Check sheet for the drawn part. Datum: minimum x, y, z corner. Units: mm. A direction names the side the tool comes from. Round coordinates to 2 decimals unless told otherwise and drop trailing zeros. Loops run counter-clockwise (first coordinate to the right, second up) from the corner with the lowest first, then second, coordinate; pieces in that order, holes last. Notation, with made-up numbers: (64, -7) - (111, -7) arc R16 cw to (111, 19) - close; hole circle Ø2 at (-38, 64.25). An arc over 180 degrees is marked (long way). Use CSV: the item, a comma, the result in double quotes.
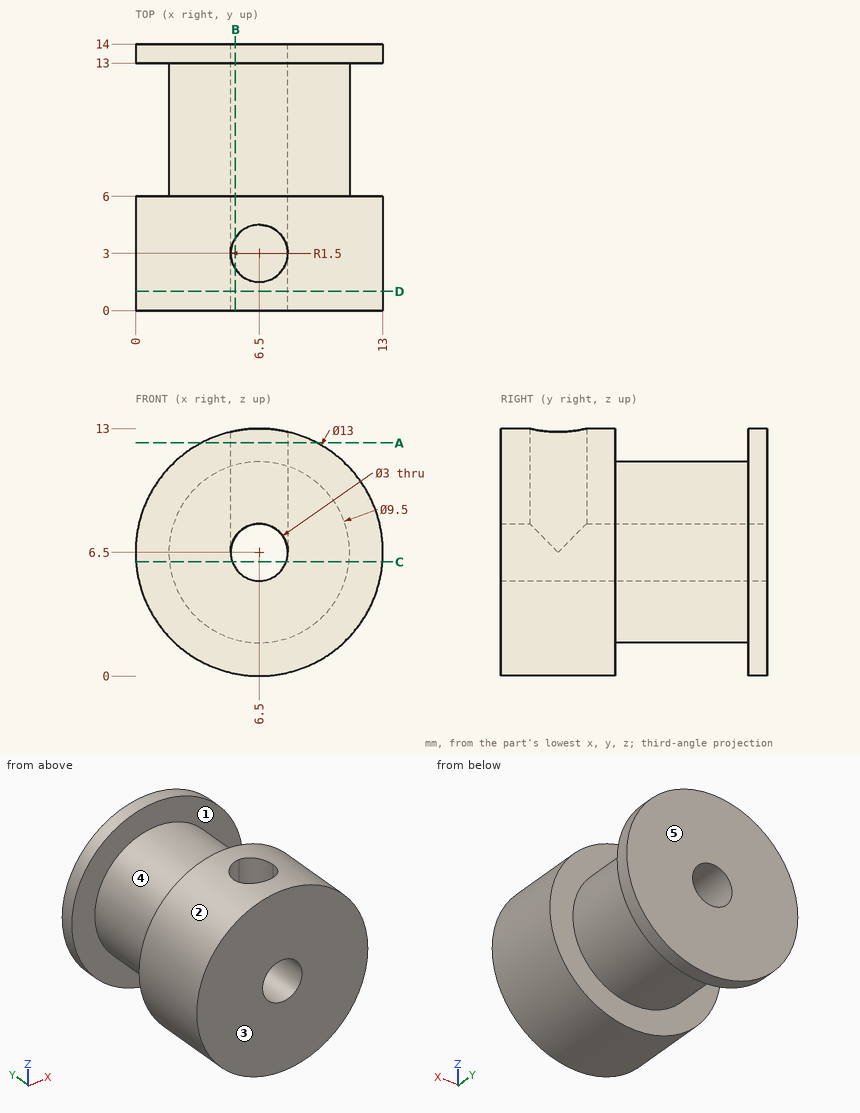
1) Gauge pin test, flat ends, axial feed: pin 1 Ø1.5 at (y, z) = (10.5, 8.5) entering from -X; pin 2 Ø1 at (y, z) = (6, 5.5) entering from -X. Record the tip position at first contact, or that the pin passes through.
Returned:
pin 1,"stops at x = 1.92"
pin 2,"stops at x = 0.02"
2) Cross-section at B-B, the plane x = 5.25. Record the cut outline in (y, z).
Returned:
outline,"(0, 0.12) - (6, 0.12) - (6, 1.92) - (13, 1.92) - (13, 0.12) - (14, 0.12) - (14, 5.67) - (0, 5.67) - close; (0, 7.33) - (2.17, 7.33) - (2.17, 12.88) - (0, 12.88) - close; (3.83, 7.33) - (14, 7.33) - (14, 12.88) - (13, 12.88) - (13, 11.08) - (6, 11.08) - (6, 12.88) - (3.83, 12.88) - close"
3) Cross-section at C-C, the plane z = 6. Record the cut outline in (x, y), then the cut area to 3 significant figures.
Returned:
outline,"(0.02, 0) - (5.09, 0) - (5.09, 14) - (0.02, 14) - (0.02, 13) - (1.78, 13) - (1.78, 6) - (0.02, 6) - close; (7.91, 0) - (12.98, 0) - (12.98, 6) - (11.22, 6) - (11.22, 13) - (12.98, 13) - (12.98, 14) - (7.91, 14) - close"
area,"117 mm²"
4) Cross-section at A-A, the plane z = 12.25. Record the cut outline in (x, y), then the cut area to 3 significant figures.
Returned:
outline,"(3.47, 0) - (9.53, 0) - (9.53, 6) - (3.47, 6) - close; (3.47, 13) - (9.53, 13) - (9.53, 14) - (3.47, 14) - close; hole circle Ø3 at (6.5, 3)"
area,"35.4 mm²"
5) Mould release check, pull along Y, two halves, no side actions. Record for the marked faces 3, 4 and 5: +Y half, -Y half, draft (parallel to the pull), parting line (faces both ways), or undercut.
Returned:
face 3,"-Y half"
face 4,"undercut"
face 5,"+Y half"
6) Access from +Z, -Z, +X, -X, +Y, -Y to the whole of each face (thin tool, end or side, straight path). Record for the marked faces 1 and 2.
Returned:
face 1,"none"
face 2,"+Y, -Y"
7) Cross-section at D-D, the plane y = 1. Record the cut outline in (x, z), then the cut area to 3 significant figures.
Returned:
outline,"circle Ø13 at (6.5, 6.5); hole circle Ø3 at (6.5, 6.5)"
area,"126 mm²"
8) Thickness scan on probe 1 along X at (y, z) = (4.75, 6.5); probe 2 along X at (y, z) = (6.5, 6.5); probe 3 along Y at (x, z) = (9.5, 11.25). Record the ranges inside material, lowest first. Write a range as [from, to].
Returned:
probe 1,"x = [0, 5], [8, 13]"
probe 2,"x = [1.75, 5], [8, 11.25]"
probe 3,"y = [0, 6], [13, 14]"
